Geometry check sheet. Reference: the model listing, model coordinates, mm. A direction names the side the tool comes from. Round coordinates to 2 decimals unless told otherwise and drop trailing zeros. Write each loop counter-clockwise with the first axis right and the second up, starting at its lowest first coordinate (ties: lowest second). Pieces come first, ordered by that corner, then holes.
Item 1: Scan lines: probe 1 along Y at (x, z) = (0.5, 7); probe 2 along X at (y, z) = (-18.5, 10.25); probe 3 along X at (y, z) = (-1.5, 12.5). Record each from-to range of solid material in increasing order.
Item 2: Cross-section at A-A (z = 12.5). Enter the section's corners in (x, y), then the cut area to 3 significant figures.
Item 3: Cross-section at C-C (x = 10.5). Enter the section's corners in (y, z), then the cut area to 3 significant figures.
Item 4: Cross-section at D-D (x = 0). Enter the section's corners in (y, z), then the cut area to 3 significant figures.
Item 5: Cross-section at B-B (y = 0). Enter the section's corners in (x, z).
Item 6: Draft check along Z on faces 1 (the face through (-24, -16.743, 10.728)), 2 (the face through (0, -23, 5)), 3 (the face through (-22.78, -13.11, 13.93)). Enter one of: pulls with the +Z half, pulls with the -Z half, needs draft (parallel to the pull), parting line crosses it, or undercut.
Item 7: Access from +Z, -Z, +X, -X, +Y, -Y to the whole of each face (thin tool, end or side, straight path). Record for faces 4 (the face through (20.917, -14.963, 10.728)), 5 (the face through (-2.5, 26, 11)), 6 (the face through (17.447, 9.775, 12.395)).
Item 8: Depth check by flat-ended pin: P1, Ø2, axis at x = -27.5, y = 19.5, coming from the +Z side; P2, Ø1.5, axis at x = -25, z = 2, coming from the -Y side; P3, Ø1.5, axis at x = 17, z = 9, coming from the -Y side. Enter the tip coordinate at first touch or a pass-through.
from build123d import *

# Parameters (mm, degrees)
SKETCH2_R           = 35
SKETCH2_R_2         = 15
BOSS_EXTRUDE1_DEPTH = 5
SKETCH3_R           = 19.99897621
SKETCH3_R_2         = 15
BOSS_EXTRUDE3_DEPTH = 15
CUT_EXTRUDE1_REACH  = 57.057
SKETCH4_R           = 1.8
CIRPATTERN1_COUNT   = 3


with BuildPart() as part:
    # Sketch2 → Boss-Extrude1 (new body)
    with BuildSketch(Plane.XY):
        Circle(SKETCH2_R)
        Circle(SKETCH2_R_2, mode=Mode.SUBTRACT)
    extrude(amount=BOSS_EXTRUDE1_DEPTH)

    # Sketch3 → Boss-Extrude3 (add)
    # profile 1 of 4: a face of its own
    with BuildSketch(Plane.XY.offset(5)):
        Circle(SKETCH3_R)
        Circle(SKETCH3_R_2, mode=Mode.SUBTRACT)
    # profile 2 of 4: a face of its own
    with BuildSketch(Plane.XY.offset(5)):
        with BuildLine():
            Line((-2.5, 34.910600109), (-2.5, 19.84210295))
            ThreePointArc((-2.5, 19.84210295), (0, 19.99897621), (2.5, 19.84210295))
            Line((2.5, 19.84210295), (2.5, 34.910600109))
            ThreePointArc((2.5, 34.910600109), (0, 35), (-2.5, 34.910600109))
        make_face()
    # profile 3 of 4: a face of its own
    with BuildSketch(Plane.XY.offset(5)):
        with BuildLine():
            ThreePointArc((18.433765219, -7.755987965), (17.319621448, -9.999488105), (15.933765219, -12.086114984))
            Line((15.933765219, -12.086114984), (28.983466556, -19.620363564))
            ThreePointArc((28.983466556, -19.620363564), (30.310889132, -17.5), (31.483466556, -15.290236545))
            Line((31.483466556, -15.290236545), (18.433765219, -7.755987965))
        make_face()
    # profile 4 of 4: a face of its own
    with BuildSketch(Plane.XY.offset(5)):
        with BuildLine():
            Line((-28.983466556, -19.620363564), (-15.933765219, -12.086114984))
            ThreePointArc((-15.933765219, -12.086114984), (-17.319621448, -9.999488105), (-18.433765219, -7.755987965))
            Line((-18.433765219, -7.755987965), (-31.483466556, -15.290236545))
            ThreePointArc((-31.483466556, -15.290236545), (-30.310889132, -17.5), (-28.983466556, -19.620363564))
        make_face()
    extrude(amount=BOSS_EXTRUDE3_DEPTH)

    # Sketch4 → Cut-Extrude1 (cut, up to next)
    with BuildSketch(Plane(origin=(2.5, 0, 0), x_dir=(0, 0, -1), z_dir=(1, 0, 0)), mode=Mode.PRIVATE) as cut_extrude1_sk1:
        with Locations((-12.5, 27.376351529)):
            Circle(SKETCH4_R)
    cut_extrude1_tool1 = extrude(cut_extrude1_sk1.sketch, amount=-CUT_EXTRUDE1_REACH, mode=Mode.PRIVATE) & part.part
    cut_extrude1 = cut_extrude1_tool1.solids().sort_by_distance((2.5, 27.376352, 12.5))[0]
    add(cut_extrude1, mode=Mode.SUBTRACT)

    # CirPattern1: Cut-Extrude1 ×3 about axis
    cirpattern1_axis = Axis((0, 0, 5), (0, 0, -1))
    for i in range(1, CIRPATTERN1_COUNT):
        add(cut_extrude1.rotate(cirpattern1_axis, i * 360 / CIRPATTERN1_COUNT), mode=Mode.SUBTRACT)


solid = part.part
Resolved:
1. probe 1: y = -19.99 to -14.99, 14.99 to 35
1. probe 2: x = -29.71 to -27.04, -7.6 to 7.6, 27.04 to 29.71
1. probe 3: x = -19.94 to -14.92, 14.92 to 19.94
2. outline: (-31.48, -15.29) arc R35 ccw to (-28.98, -19.62) - (-24.02, -16.75) - (-26.52, -12.42) - close; (-23.4, -10.62) - (-20.9, -14.95) - (-15.93, -12.09) arc R20 ccw to (15.93, -12.09) - (20.9, -14.95) - (23.4, -10.62) - (18.43, -7.76) arc R20 ccw to (2.5, 19.84) - (2.5, 25.58) - (-2.5, 25.58) - (-2.5, 19.84) arc R20 ccw to (-18.43, -7.76) - close; (-2.5, 29.18) - (2.5, 29.18) - (2.5, 34.91) arc R35 ccw to (-2.5, 34.91) - close; (24.02, -16.75) - (28.98, -19.62) arc R35 ccw to (31.48, -15.29) - (26.52, -12.42) - close; hole circle Ø30 at (0, 0)
2. area: 721 mm2
3. outline: (-33.39, 0) - (-10.71, 0) - (-10.71, 20) - (-17.02, 20) - (-17.02, 5) - (-33.39, 5) - close; (10.71, 0) - (33.39, 0) - (33.39, 5) - (17.02, 5) - (17.02, 20) - (10.71, 20) - close
3. area: 416 mm2
4. outline: (-35, 0) - (-15, 0) - (-15, 20) - (-20, 20) - (-20, 5) - (-35, 5) - close; (15, 0) - (35, 0) - (35, 20) - (15, 20) - close; hole circle Ø3.6 at (27.38, 12.5)
4. area: 565 mm2
5. outline: (-35, 0) - (-15, 0) - (-15, 20) - (-20, 20) - (-20, 5) - (-35, 5) - close; (15, 0) - (35, 0) - (35, 5) - (20, 5) - (20, 20) - (15, 20) - close
6. face 1: needs draft
6. face 2: pulls with the +Z half
6. face 3: undercut
7. face 4: +Z, -Y
7. face 5: +Z, -X, +Y
7. face 6: +Z, +X
8. P1: stops at z = 5
8. P2: stops at y = -25.24
8. P3: stops at y = -13.13
